from build123d import *

# Parameters (mm, degrees)
SKETCH1_W           = 1991
SKETCH1_H           = 1625
BOSS_EXTRUDE1_DEPTH = 1
CUT_EXTRUDE1_DEPTH  = 2789.8673629


with BuildPart() as part:
    # Sketch1 → Boss-Extrude1 (new body)
    with BuildSketch(Plane.XY):
        with Locations((995.5, 812.5)):
            Rectangle(SKETCH1_W, SKETCH1_H)
    extrude(amount=BOSS_EXTRUDE1_DEPTH)

    # Sketch2 → Cut-Extrude1 (cut, through all)
    with BuildSketch(Plane(origin=(259.963517843, -561.616762327, 1), x_dir=(1, 0, 0), z_dir=(0, 0, 1))):
        with BuildLine():
            Line((1498.845356152, 2093.616540003), (1224.605356152, 1618.616540003))
            ThreePointArc((1224.605356152, 1618.616540003), (1224.605548691, 1500.616651165), (1326.796482157, 1441.616762327))
            Line((1326.796482157, 1441.616762327), (1551.036482157, 1441.616762327))
            ThreePointArc((1551.036482157, 1441.616762327), (1669.830421397, 1490.822823088), (1719.036482157, 1609.616762327))
            Line((1719.036482157, 1609.616762327), (1719.036482157, 2034.616762327))
            ThreePointArc((1719.036482157, 2034.616762327), (1631.577005494, 2148.596043051), (1498.845356152, 2093.616540003))
        make_face()
        with BuildLine():
            Line((-247.963517843, 1984.616762327), (-247.963517843, 1559.616762327))
            ThreePointArc((-247.963517843, 1559.616762327), (-160.504041179, 1445.637481603), (-27.772391837, 1500.616984652))
            Line((-27.772391837, 1500.616984652), (246.467608163, 1975.616984652))
            ThreePointArc((246.467608163, 1975.616984652), (246.467415624, 2093.61687349), (144.276482157, 2152.616762327))
            Line((144.276482157, 2152.616762327), (-79.963517843, 2152.616762327))
            ThreePointArc((-79.963517843, 2152.616762327), (-198.757457082, 2103.410701567), (-247.963517843, 1984.616762327))
        make_face()
    extrude(amount=-CUT_EXTRUDE1_DEPTH, mode=Mode.SUBTRACT)


solid = part.part
The model under review builds one solid part; all positions refer to its coordinate system, in mm. A direction names the side the tool comes from. Round coordinates to 2 decimals unless told otherwise and drop trailing zeros. Write each loop counter-clockwise with the first axis right and the second up, starting at its lowest first coordinate (ties: lowest second). Pieces come first, ordered by that corner, then holes. Notation, with made-up numbers: M 33,79 L 80,79 A19 ccw 80,89 Z; hole C 28.25,-6.75 d5. An arc over 180 degrees is marked long. Use a Markdown table: item, result. Add a question column.
Q1. To check wall thickness, follow line 1 (X direction, y = 1518, z = 0.85); line 2 (X direction, y = 1152, z = 0.8); line 3 (Y direction, x = 1508, z = 0.85). State the ranges of each line that lie inside material, in increasing order.
Q2. We need section A-A, the plane x = 1710.5. State the section outline as (y, z) points, plus the area to 3 significant figures.
Q3. The part is to be moulded in two halves that separate along Y. For faces 3 (the face through (1893.62, 1586.4, 0.51)), 4 (the face through (982, 824, 0)), say which applies: pulls with the +Y half, pulls with the -Y half, needs draft (parallel to the pull), parting line crosses it, or undercut.
Q4. We need section B-B, the plane y = 1104.5. State the section outline as (x, z) points.
Q5. We need section C-C, the plane z = 0.6. State the section outline as (x, y) points, plus the area to 3 significant figures.
Q6. We need section D-D, the plane y = 1449.5. State the section outline as (x, z) points.
Q7. Machinability: for faces 1 (the face through (1483.715, 940.504, 0.507)), 2 (the face through (982, 824, 1)), which of the approach directions +Z, -Z, +X, -X, +Y, -Y give a long, thin tool a straight path to every point of the face, cutting with its end or side? Answer none if there is none.
Findings below:
| question | item | result |
|---|---|---|
| 1 | line 1 | x = 0 to 41.44, 513.32 to 1750.73, 1970.08 to 1991 |
| 1 | line 2 | x = 0 to 12, 355.17 to 1539.42, 1979 to 1991 |
| 1 | line 3 | y = 0 to 910.13, 1097.58 to 1625 |
| 2 | outline | M 0,0 L 880,0 L 880,1 L 0,1 Z; M 1448.33,0 L 1625,0 L 1625,1 L 1448.33,1 Z |
| 2 | area | 1,060 mm² |
| 3 | face 3 | undercut |
| 3 | face 4 | needs draft |
| 4 | outline | M 0,0 L 12,0 L 12,1 L 0,1 Z; M 327.74,0 L 1511.99,0 L 1511.99,1 L 327.74,1 Z; M 1979,0 L 1991,0 L 1991,1 L 1979,1 Z |
| 5 | outline | M 0,0 L 1991,0 L 1991,1625 L 0,1625 Z; hole M 12,998 A118 ccw 232.19,939 L 506.43,1414 A118 ccw 404.24,1591 L 180,1591 A168 ccw 12,1423 Z; hole M 1484.57,1057 A118 ccw 1586.76,880 L 1811,880 A168 ccw 1979,1048 L 1979,1473 A118 ccw 1758.81,1532 Z |
| 5 | area | 2,720,000 mm² |
| 6 | outline | M 0,0 L 14.1,0 L 14.1,1 L 0,1 Z; M 519.88,0 L 1711.18,0 L 1711.18,1 L 519.88,1 Z; M 1979,0 L 1991,0 L 1991,1 L 1979,1 Z |
| 7 | face 1 | +Z, -Z |
| 7 | face 2 | +Z, +X, -X, +Y, -Y |
